Build history of the part. All positions in model axes, mm. Face numbers are marked on the shaded views. Round coordinates to 2 decimals unless told otherwise and drop trailing zeros. Loops run counter-clockwise (first coordinate to the right, second up) from the corner with the lowest first, then second, coordinate; pieces in that order, holes last. Notation, with made-up numbers: (80.25, -23.75) - (98.25, -23.75) arc R27 ccw to (98.25, 8.25) - close; hole circle Ø3 at (-40, -14.75). An arc over 180 degrees is marked (long way). Use a Markdown table: item, result.
from build123d import *

# Parameters (mm, degrees)
BOSS_EXTRUDE1_DEPTH = 1.3
SKETCH5_R           = 5
CUT_EXTRUDE1_DEPTH  = 28


with BuildPart() as part:
    # Sketch2 → Boss-Extrude1 (new body)
    with BuildSketch(Plane.XY):
        with BuildLine():
            Line((-20.5, -0.65), (-13.5, -0.65))
            ThreePointArc((-13.5, -0.65), (-12.333273811, -0.166726189), (-11.85, 1))
            Line((-11.85, 1), (-11.85, 7))
            ThreePointArc((-11.85, 7), (-11, 7.85), (-10.15, 7))
            Line((-10.15, 7), (-10.15, 0))
            Line((-10.15, 0), (-10.15, -7))
            ThreePointArc((-10.15, -7), (-8, -9.15), (-5.85, -7))
            Line((-5.85, -7), (-5.85, 0))
            Line((-5.85, 0), (-5.85, 7))
            ThreePointArc((-5.85, 7), (-5, 7.85), (-4.15, 7))
            Line((-4.15, 7), (-4.15, 0))
            Line((-4.15, 0), (-4.15, -7))
            ThreePointArc((-4.15, -7), (-2, -9.15), (0.15, -7))
            Line((0.15, -7), (0.15, 0))
            Line((0.15, 0), (0.15, 7))
            ThreePointArc((0.15, 7), (1, 7.85), (1.85, 7))
            Line((1.85, 7), (1.85, 0))
            Line((1.85, 0), (1.85, -7))
            ThreePointArc((1.85, -7), (4, -9.15), (6.15, -7))
            Line((6.15, -7), (6.15, -1))
            ThreePointArc((6.15, -1), (6.252512627, -0.752512627), (6.5, -0.65))
            Line((6.5, -0.65), (13.5, -0.65))
            ThreePointArc((13.5, -0.65), (14.15, 0), (13.5, 0.65))
            Line((13.5, 0.65), (6.5, 0.65))
            ThreePointArc((6.5, 0.65), (5.333273811, 0.166726189), (4.85, -1))
            Line((4.85, -1), (4.85, -7))
            ThreePointArc((4.85, -7), (4, -7.85), (3.15, -7))
            Line((3.15, -7), (3.15, 0))
            Line((3.15, 0), (3.15, 7))
            ThreePointArc((3.15, 7), (1, 9.15), (-1.15, 7))
            Line((-1.15, 7), (-1.15, 0))
            Line((-1.15, 0), (-1.15, -7))
            ThreePointArc((-1.15, -7), (-2, -7.85), (-2.85, -7))
            Line((-2.85, -7), (-2.85, 0))
            Line((-2.85, 0), (-2.85, 7))
            ThreePointArc((-2.85, 7), (-5, 9.15), (-7.15, 7))
            Line((-7.15, 7), (-7.15, 0))
            Line((-7.15, 0), (-7.15, -7))
            ThreePointArc((-7.15, -7), (-8, -7.85), (-8.85, -7))
            Line((-8.85, -7), (-8.85, 0))
            Line((-8.85, 0), (-8.85, 7))
            ThreePointArc((-8.85, 7), (-11, 9.15), (-13.15, 7))
            Line((-13.15, 7), (-13.15, 1))
            ThreePointArc((-13.15, 1), (-13.252512627, 0.752512627), (-13.5, 0.65))
            Line((-13.5, 0.65), (-20.5, 0.65))
            ThreePointArc((-20.5, 0.65), (-21.15, 0), (-20.5, -0.65))
        make_face()
    extrude(amount=BOSS_EXTRUDE1_DEPTH)

    # Sketch3 → Revolve1 (revolve)
    with BuildSketch(Plane(origin=(0, 0, 0), x_dir=(1, 0, 0), z_dir=(0, 1, 0)), mode=Mode.PRIVATE) as revolve1_sk:
        Polygon((-20.5, -1.3), (-25.5, -1.3), (-26.5, 2.7), (-26.5, 28.7), (-20.5, 28.7), align=None)
    revolve(revolve1_sk.sketch.rotate(Axis((-20.5, 0, 1.3), (0, 0, -1)), 187.469592391), axis=Axis((-20.5, 0, 1.3), (0, 0, -1)))

    # Sketch4 → Revolve2 (revolve)
    with BuildSketch(Plane(origin=(0, 0, 0), x_dir=(1, 0, 0), z_dir=(0, 1, 0)), mode=Mode.PRIVATE) as revolve2_sk:
        Polygon((13.5, -1.3), (18.5, -1.3), (19.5, 2.7), (19.5, 28.7), (13.5, 28.7), align=None)
    revolve(revolve2_sk.sketch.rotate(Axis((13.5, 0, 1.3), (0, 0, -1)), 172.988663576), axis=Axis((13.5, 0, 1.3), (0, 0, -1)))

    # Sketch5 → Cut-Extrude1 (cut)
    with BuildSketch(Plane(origin=(0, 0, -28.7), x_dir=(-1, 0, 0), z_dir=(0, 0, -1))):
        with Locations((20.5, 0)):
            Circle(SKETCH5_R)
        with Locations((-13.5, 0)):
            Circle(SKETCH5_R)
    extrude(amount=-CUT_EXTRUDE1_DEPTH, mode=Mode.SUBTRACT)


solid = part.part
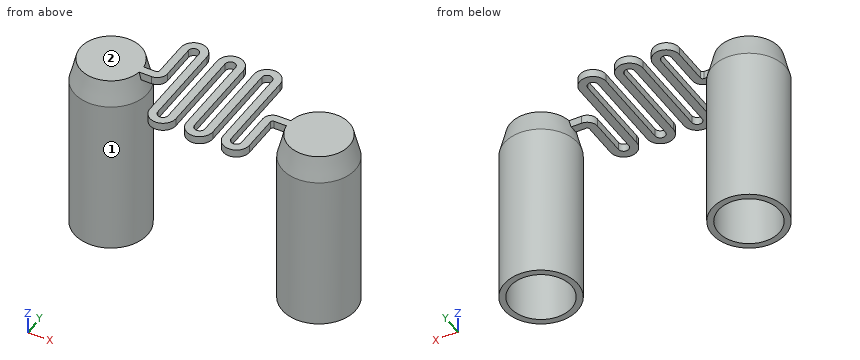
Q1. Cut at C-C, the plane y = 0. Count the separate pieces of the cut face and the enclosed holes in it, plus the area to 3 significant figures.
Results found:
| item | result |
|---|---|
| separate pieces | 7 |
| enclosed holes | 0 |
| area | 169 mm2 |
Q2. Drop flat-ended pins along their axis: pin 1 (1.4 mm diameter, centred on y = -0.5, z = 0.5, fed in from -X); pin 2 (1 mm diameter, centred on y = 1.5, z = 0.5, fed in from -X); pin 3 (0.6 mm diameter, centred on y = -3, z = 0.5, fed in from +X); pin 4 (1.5 mm diameter, centred on x = 6, z = -24, fed in from -Y). Give the stop position or say it passes through.
Results found:
| item | result |
|---|---|
| pin 1 | stops at x = -25.86 |
| pin 2 | stops at x = -25.66 |
| pin 3 | stops at x = 17.96 |
| pin 4 | passes through |
Q3. Probe line 1 (X direction, y = 0.25, z = -11.5); line 2 (Y direction, x = -20.5, z = -17.5); line 3 (X direction, y = 3.75, z = -22). List the from-to ranges inside material, lowest first.
Results found:
| item | result |
|---|---|
| line 1 | x = -26.49 to -25.49, -15.51 to -14.51, 7.51 to 8.51, 18.49 to 19.49 |
| line 2 | y = -6 to -5, 5 to 6 |
| line 3 | x = -25.18 to -23.81, -17.19 to -15.82, 8.82 to 10.19, 16.81 to 18.18 |
Q4. Cut at A-A, the plane x = 13.5. List the corners of the cut face in (y, z), plus the area to 3 significant figures.
Results found:
| item | result |
|---|---|
| outline | (-6, -28.7) - (-5, -28.7) - (-5, -0.7) - (5, -0.7) - (5, -28.7) - (6, -28.7) - (6, -2.7) - (5, 1.3) - (-5, 1.3) - (-6, -2.7) - close |
| area | 76.0 mm2 |
Q5. Cut at B-B, the plane z = -20. List the corners of the cut face in (x, y), plus the area to 3 significant figures.
Results found:
| item | result |
|---|---|
| outline | circle Ø12 at (-20.5, 0); circle Ø12 at (13.5, 0); hole circle Ø10 at (-20.5, 0); hole circle Ø10 at (13.5, 0) |
| area | 69.1 mm2 |
Q6. Pull direction X, two halves, no side cores. Call the marked faces 1 and 2: pulls with the +X half, pulls with the -X half, needs draft (parallel to the pull), parting line crosses it, or undercut.
Results found:
| item | result |
|---|---|
| face 1 | undercut |
| face 2 | needs draft |
